For this review, take the finished solid that the model builds, in its own axes (mm). A direction names the side the tool comes from. Round coordinates to 2 decimals unless told otherwise and drop trailing zeros. Loops run counter-clockwise (first coordinate to the right, second up) from the corner with the lowest first, then second, coordinate; pieces in that order, holes last. Notation, with made-up numbers: (34.5, -13.75) -> (56.5, -13.75) arc R18 cw to (56.5, -9.75) -> close; hole circle Ø10 at (62, 26). An arc over 180 degrees is marked (long way). Use one line per item in the form item = value. Start each with the question number.
Autodesk Fusion 360 part; units mm, degrees
sketch "Sketch1" plane through (0, 0, 0) normal (0, 0, 1) x (1, 0, 0)
  line L0 (28, -6.5) -> (-28, -6.5)
  line L1 (-30, -4.5) -> (-30, 4.5)
  line L2 (-28, 6.5) -> (28, 6.5)
  line L3 (30, 4.5) -> (30, -4.5)
  line L4 (30, -6.5) -> (-30, 6.5) construction
  line L5 (-30, -6.5) -> (30, 6.5) construction
  line L6 (0, 0) -> (20, 0) construction
  line L7 (0, 0) -> (-20, 0) construction
  arc A0 (30, 4.5) -> (28, 6.5) centre (28, 4.5) ccw
  arc A1 (28, -6.5) -> (30, -4.5) centre (28, -4.5) ccw
  arc A2 (-30, -4.5) -> (-28, -6.5) centre (-28, -4.5) ccw
  arc A3 (-28, 6.5) -> (-30, 4.5) centre (-28, 4.5) ccw
  circle A4 centre (20, 0) radius 3
  circle A5 centre (-20, 0) radius 3
  dimension "d1" = 60
  dimension "d2" = 13
  dimension "d3" = 20
  dimension "d4" = 2
  dimension "d5" = 20
  dimension "d6" = 6
  dimension "d7" = 6
extrude "Extrude1" add sketch "Sketch1" along normal blind 3
sketch "Sketch2" plane through (0, 0, 3) normal (0, 0, 1) x (-1, 0, 0)
  circle A0 centre (-20, 0) radius 3
  circle A1 centre (20, 0) radius 3
  arc A2 (-30, -4.5) -> (-28, -6.5) centre (-28, -4.5) ccw
  line L0 (-28, -6.5) -> (28, -6.5)
  arc A3 (28, -6.5) -> (30, -4.5) centre (28, -4.5) ccw
  line L1 (30, -4.5) -> (30, 4.5)
  arc A4 (30, 4.5) -> (28, 6.5) centre (28, 4.5) ccw
  line L2 (28, 6.5) -> (-28, 6.5)
  arc A5 (-28, 6.5) -> (-30, 4.5) centre (-28, 4.5) ccw
  line L3 (-30, 4.5) -> (-30, -4.5)
  line L4 (-12.5, 6.5) -> (12.5, 6.5)
  line L5 (12.5, 6.5) -> (12.5, -6.5)
  line L6 (12.5, -6.5) -> (-12.5, -6.5)
  line L7 (-12.5, -6.5) -> (-12.5, 6.5)
  line L8 (-12.5, 6.5) -> (12.5, -6.5) construction
  line L9 (12.5, 6.5) -> (-12.5, -6.5) construction
  line L10 (0, 0) -> (-6.5, 0) construction
  line L11 (0, 0) -> (6.5, 0) construction
  dimension "d10" = 25
  dimension "d11" = 6.5
  dimension "d12" = 6.5
extrude "Extrude2" add sketch "Sketch2" along normal blind 10 contours L0 L2 L4 L5 L6 L7
sketch "Sketch3" plane through (0, 0, 0) normal (0, 0, 1) x (-1, 0, 0)
  line L0 (-12.5, -6.5) -> (12.5, -6.5)
  line L1 (12.5, -6.5) -> (12.5, 6.5)
  line L2 (12.5, 6.5) -> (-12.5, 6.5)
  line L3 (-12.5, 6.5) -> (-12.5, -6.5)
  line L4 (0, 0) -> (-6.5, 0) construction
  line L5 (0, 0) -> (6.5, 0) construction
  circle A0 centre (-6.5, 0) radius 2.6
  line L6 (0, 0) -> (0, -2) construction
  circle A1 centre (6.5, 0) radius 2.6
  circle A2 centre (-20, 0) radius 3
  circle A3 centre (20, 0) radius 3
  arc A4 (-30, -4.5) -> (-28, -6.5) centre (-28, -4.5) ccw
  line L7 (-30, -4.5) -> (-30, 4.5)
  arc A5 (-28, 6.5) -> (-30, 4.5) centre (-28, 4.5) ccw
  line L8 (-28, 6.5) -> (28, 6.5)
  arc A6 (30, 4.5) -> (28, 6.5) centre (28, 4.5) ccw
  line L9 (30, 4.5) -> (30, -4.5)
  arc A7 (28, -6.5) -> (30, -4.5) centre (28, -4.5) ccw
  line L10 (28, -6.5) -> (-28, -6.5)
  dimension "d15" = 6.5
  dimension "d16" = 6.5
  dimension "d17" = 5.2
  dimension "d18" = 2
hole "Hole1" at (6.5, 0, 0) at (-6.5, 0, 0) direction (0, 0, 1) diameter 5.2 depth 13 tip angle 90 countersink diameter 5.72 countersink angle 90
Item 1: Take a section at D-D on z = 9. Give the boundary of the cut face in (x, y), plus the area to 3 significant figures.
Item 2: Take a section at C-C on x = 6.5. Give the boundary of the cut face in (y, z), plus the area to 3 significant figures.
Item 3: Draft analysis for pull direction X (two halves, no side actions). For faces 4 (the flat face through (-23.3, 0.1, 3)), 5 (the cylindrical face through (-23, 0, 1)), 6 (the flat face through (-30, 0, 1)), state which applies: +X half, -X half, draft (parallel to the pull), parting line (faces both ways), or undercut.
Item 4: Take a section at B-B on y = -3.75. Give the boundary of the cut face in (x, z).
Item 5: Take a section at A-A on x = 20. Give the boundary of the cut face in (y, z), plus the area to 3 significant figures.
Item 6: Wall thickness on line 1 (X direction, y = -0.25, z = 2); line 2 (Y direction, x = -20, z = 1.6); line 3 (Y direction, x = 6.5, z = 8): over which ranges is each line inside the solid? List them lowest first.
Item 7: Machinability: for faces 1 (the flat face through (-12.5, 0, 8)), 2 (the cylindrical face through (3.922, -0.338, 6.719)), 3 (the flat face through (12.5, 0, 8)), which of the approach directions +Z, -Z, +X, -X, +Y, -Y give a long, thin tool a straight path to every point of the face, cutting with its end or side? Answer none if there is none.
Item 8: For P1, Ø4, axis at x = -6.5, y = 0, coming from the +Z side; P2, Ø2, axis at y = 0, z = 6.5, coming from the +X side; P3, Ø1.5, axis at y = -4, z = 11, coming from the -X side; P4, Ø1.5, axis at x = -23.5, y = -1, coming from the +Z side, all flat-tipped, find the tip position at first contact; note any pin that passes through.
Results:
q1.outline = (-12.5, -6.5) -> (12.5, -6.5) -> (12.5, 6.5) -> (-12.5, 6.5) -> close; hole circle Ø5.2 at (-6.5, 0); hole circle Ø5.2 at (6.5, 0)
q1.area = 283 mm2
q2.outline = (-6.5, 0) -> (-2.86, 0) -> (-2.6, 0.26) -> (-2.6, 13) -> (-6.5, 13) -> close; (2.6, 0.26) -> (2.86, 0) -> (6.5, 0) -> (6.5, 13) -> (2.6, 13) -> close
q2.area = 101 mm2
q3.face_4 = draft
q3.face_5 = undercut
q3.face_6 = -X half
q4.outline = (-30, 0) -> (30, 0) -> (30, 3) -> (12.5, 3) -> (12.5, 13) -> (-12.5, 13) -> (-12.5, 3) -> (-30, 3) -> close
q5.outline = (-6.5, 0) -> (-3, 0) -> (-3, 3) -> (-6.5, 3) -> close; (3, 0) -> (6.5, 0) -> (6.5, 3) -> (3, 3) -> close
q5.area = 21.0 mm2
q6.line_1 = -30 to -22.99, -17.01 to -9.09, -3.91 to 3.91, 9.09 to 17.01, 22.99 to 30
q6.line_2 = -6.5 to -3, 3 to 6.5
q6.line_3 = -6.5 to -2.6, 2.6 to 6.5
q7.face_1 = +Z, -X, +Y, -Y
q7.face_2 = +Z, -Z
q7.face_3 = +Z, +X, +Y, -Y
q8.P1 = through
q8.P2 = 12.5
q8.P3 = -12.5
q8.P4 = 3
